Verification items for the finished model (mm, model axes). Face numbers are marked on the shaded views. A direction names the side the tool comes from. Give positions to 0.01 mm unless a question says otherwise; leave off trailing zeros. Loops run counter-clockwise (first coordinate to the right, second up) from the corner with the lowest first, then second, coordinate; pieces in that order, holes last. Notation, with made-up numbers: (-14, 82) - (44, 82) arc R17 cw to (44, 100) - close; hole circle Ø10 at (20, 52). An arc over 180 degrees is marked (long way). One line per item, written item: value. Start each with the question number.
1. Sectioned sample at B-B (z = 0). Record the cut outline in (x, y), plus the area to 3 significant figures.
2. Sectioned sample at A-A (y = 3.5). Record the cut outline in (x, z).
3. Sectioned sample at D-D (y = -1). Record the cut outline in (x, z).
4. Access from +Z, -Z, +X, -X, +Y, -Y to the whole of each face (thin tool, end or side, straight path). Record for the marked faces 1 and 2.
5. Scan lines: L1, parallel to Y at x = 1.85, z = 0.1; L2, parallel to Y at x = -0.5, z = 0.5; L3, parallel to Z at x = 1.05, y = 3.5. Record each from-to range of solid material in increasing order. Write a range as [from, to].
6. Sectioned sample at C-C (x = -0.35). Record the cut outline in (y, z).
7. Mould release check, pull along X, two halves, no side actions. Record for the marked faces 3, 4, 5 and 6: pulls with the +X half, pulls with the -X half, needs draft (parallel to the pull), parting line crosses it, or undercut.
8. Gauge pin test, flat ends, axial feed: pin 1 (3 mm diameter, centred on y = -3.5, z = 2, fed in from +X); pin 2 (3 mm diameter, centred on y = 3, z = 0.5, fed in from -X); pin 3 (0.8 mm diameter, centred on x = 0.5, z = -0.5, fed in from +Y). Record the tip position at first contact, or that the pin passes through.
from build123d import *

# Parameters (mm, degrees)
EXTRUSION1_DEPTH        = 5
ESQUISSE2_R             = 1.25
EXTRUSION2_DEPTH        = 5
ESQUISSE3_R             = 1.25
ENL_V_MAT_EXTRU_2_DEPTH = 4


with BuildPart() as part:
    # Esquisse1 → Extrusion1 (new body)
    with BuildSketch(Plane(origin=(0, 0, 0), x_dir=(1, 0, 0), z_dir=(0, 1, 0))):
        Polygon((2.424630573, 1.56668437), (-0.144473178, 2.883133856), (-2.569103751, 1.316449486), (-2.424630573, -1.56668437), (0.144473178, -2.883133856), (2.569103751, -1.316449486), align=None)
    extrude(amount=EXTRUSION1_DEPTH)

    # Esquisse2 → Extrusion2 (add)
    with BuildSketch(Plane.XZ):
        with Locations(Location((0, 0, 0), (0, 0, 270))):  # turned: the seam where the file's is
            Circle(ESQUISSE2_R)
    extrude(amount=EXTRUSION2_DEPTH)

    # Esquisse3 → Enlèv. mat.-Extru.2 (cut)
    with BuildSketch(Plane(origin=(0, 5, 0), x_dir=(-1, 0, 0), z_dir=(0, 1, 0))):
        with Locations(Location((0, 0, 0), (0, 0, 270))):  # turned: the seam where the file's is
            Circle(ESQUISSE3_R)
    extrude(amount=-ENL_V_MAT_EXTRU_2_DEPTH, mode=Mode.SUBTRACT)


solid = part.part
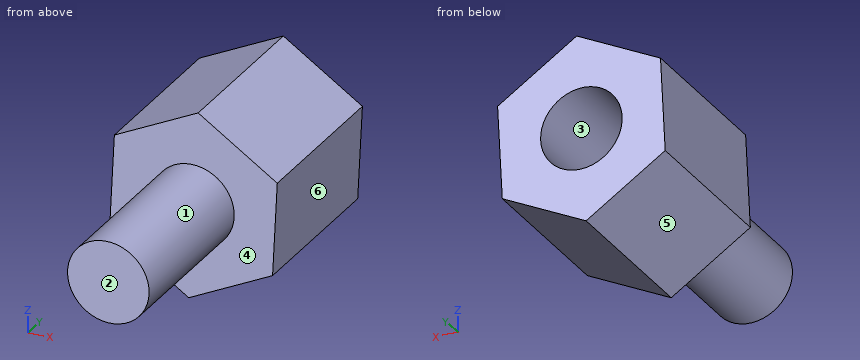
Results are:
1. outline: (-2.5, 0) - (-1.25, 0) - (-1.25, -5) - (1.25, -5) - (1.25, 0) - (2.5, 0) - (2.5, 5) - (1.25, 5) - (1.25, 1) - (-1.25, 1) - (-1.25, 5) - (-2.5, 5) - close
1. area: 27.5 mm^2
2. outline: (-2.57, -1.32) - (-0.14, -2.88) - (2.42, -1.57) - (2.57, 1.32) - (0.14, 2.88) - (-2.42, 1.57) - close; hole circle Ø2.5 at (0, 0)
3. outline: circle Ø2.5 at (0, 0)
4. face 1: -Y
4. face 2: +Z, -Z, +X, -X, -Y
5. L1: y = [0, 5]
5. L2: y = [-5, 1]
5. L3: z = [-2.27, -0.68], [0.68, 2.3]
6. outline: (-5, -1.2) - (0, -1.2) - (0, -2.75) - (5, -2.75) - (5, -1.2) - (1, -1.2) - (1, 1.2) - (5, 1.2) - (5, 2.63) - (0, 2.63) - (0, 1.2) - (-5, 1.2) - close
7. face 3: undercut
7. face 4: needs draft
7. face 5: pulls with the -X half
7. face 6: pulls with the +X half
8. pin 1: stops at x = 1.15
8. pin 2: stops at x = -2.55
8. pin 3: stops at y = 1
